Build history of the part. All positions in model axes, mm. A direction names the side the tool comes from. Give positions to 0.01 mm unless a question says otherwise; leave off trailing zeros. Order: outer loops, then holes, each group sorted by start corner. A loop starts at its lowest first (then second) coordinate and runs counter-clockwise, first axis right, second up. Notation, with made-up numbers: (-21, -26) -> (16, -26) arc R29 ccw to (16, 10) -> close; hole circle Ø10 at (-33.5, 86). An arc over 180 degrees is marked (long way). One line per item, written item: value. Start each with the question number.
(1) Saw through at A-A on z = 12. Give the cut face in (x, y), plus the area to 3 significant figures.
(2) Saw through at C-C on x = 17.5. Give the cut face in (y, z).
(3) Two-plate mould, pull along X, no slides. Class faces 1 (the flat face through (-42.25, -1, 29)), 2 (the flat face through (-1, 1, 53)), 3 (the flat face through (-1, 1, 56)), 4 (the flat face through (-39.25, 1, 27)): +X half, -X half, draft (parallel to the pull), parting line (faces both ways), or undercut.
(4) Which spindle directions (+Z, -Z, +X, -X, +Y, -Y) get a long thin tool onto all of the face, cutting with end or side? Do faces 5 (the flat face through (-52, -1, 3)), 6 (the flat face through (39.25, 1, 27)), 7 (the flat face through (0, -60, 55)), 8 (the flat face through (42.25, -1, 29)). Say none if no direction does.
(5) Saw through at B-B on y = 30. Give the cut face in (x, z).
(6) Pin check, flat tips, straight feed: pin 1 (10 mm diameter, centred on y = -19, z = 28, fed in from -X); pin 2 (10 mm diameter, centred on x = -3.5, y = 9, fed in from -Z); pin 3 (10 mm diameter, centred on x = 48, y = 18, fed in from +Z). Stop position of each tip, or through.
(7) Probe line 1 (X direction, y = 29.5, z = 34); line 2 (X direction, y = -49, z = 53.5); line 3 (Z direction, x = 25, y = -42). List the from-to ranges inside material, lowest first.
```python
from build123d import *

# Parameters (mm, degrees)
SKETCH_1_W          = 84.5
SKETCH_1_H          = 120
EXTRUDE_1_DEPTH     = 56
SKETCH_2_W          = 78.5
SKETCH_2_H          = 53
CUT_EXTRUDE_1_DEPTH = 140.00022482
SKETCH_3_W          = 3
SKETCH_3_H          = 120
EXTRUDE_2_DEPTH     = 20


with BuildPart() as part:
    # 스케치1 → 보스-돌출1 (new body)
    with BuildSketch(Plane.XY):
        Rectangle(SKETCH_1_W, SKETCH_1_H)
    extrude(amount=EXTRUDE_1_DEPTH)

    # 스케치2 → 컷-돌출1 (cut, through all)
    with BuildSketch(Plane(origin=(0, 60, 0), x_dir=(1, 0, 0), z_dir=(0, 1, 0))):
        with Locations((0, -26.5)):
            Rectangle(SKETCH_2_W, SKETCH_2_H)
    extrude(amount=-CUT_EXTRUDE_1_DEPTH, mode=Mode.SUBTRACT)

    # 스케치3 → 보스-돌출2 (add)
    with BuildSketch(Plane.ZY.offset(42.25)):
        with Locations((1.5, 0)):
            Rectangle(SKETCH_3_W, SKETCH_3_H)
    extrude_2 = extrude(amount=EXTRUDE_2_DEPTH)

    # 대칭 복사1: 보스-돌출2 across plane
    add(extrude_2.mirror(Plane(origin=(0, 0, 0), x_dir=(0, 0, 1), z_dir=(1, 0, 0))))


solid = part.part
```
Results below:
1. outline: (-42.25, -60) -> (-39.25, -60) -> (-39.25, 60) -> (-42.25, 60) -> close; (39.25, -60) -> (42.25, -60) -> (42.25, 60) -> (39.25, 60) -> close
1. area: 720 mm²
2. outline: (-60, 53) -> (60, 53) -> (60, 56) -> (-60, 56) -> close
3. face 1: -X half
3. face 2: undercut
3. face 3: draft
3. face 4: undercut
4. face 5: +Z, -X, +Y, -Y
4. face 6: -Z, +Y, -Y
4. face 7: +Z, -Z, +X, -X, -Y
4. face 8: +Z, +X, +Y, -Y
5. outline: (-62.25, 0) -> (-39.25, 0) -> (-39.25, 53) -> (39.25, 53) -> (39.25, 0) -> (62.25, 0) -> (62.25, 3) -> (42.25, 3) -> (42.25, 56) -> (-42.25, 56) -> (-42.25, 3) -> (-62.25, 3) -> close
6. pin 1: stops at x = -42.25
6. pin 2: stops at z = 53
6. pin 3: stops at z = 3
7. line 1: x = -42.25 to -39.25, 39.25 to 42.25
7. line 2: x = -42.25 to 42.25
7. line 3: z = 53 to 56
